```python
from build123d import *

# Parameters (mm, degrees)
SKETCH1_R           = 30
BOSS_EXTRUDE1_DEPTH = 17
SKETCH2_R           = 3.5
CUT_EXTRUDE1_DEPTH  = 16.5
SKETCH3_R           = 10
BOSS_EXTRUDE2_DEPTH = 1


with BuildPart() as part:
    # Sketch1 → Boss-Extrude1 (new body)
    with BuildSketch(Plane(origin=(0, 0, 0), x_dir=(1, 0, 0), z_dir=(0, 1, 0))):
        with Locations(Location((0, 0, 0), (0, 0, 270))):
            Circle(SKETCH1_R)
    extrude(amount=BOSS_EXTRUDE1_DEPTH)

    # Sketch2 → Cut-Extrude1 (cut)
    with BuildSketch(Plane.XY.offset(30)):
        with Locations((-16.875, 8.25)):
            Circle(SKETCH2_R)
        with BuildLine():
            Line((14.125, 11.75), (19.625, 11.75))
            ThreePointArc((19.625, 11.75), (23.125, 8.25), (19.625, 4.75))
            Line((19.625, 4.75), (14.125, 4.75))
            ThreePointArc((14.125, 4.75), (10.625, 8.25), (14.125, 11.75))
        make_face()
    extrude(amount=-CUT_EXTRUDE1_DEPTH, mode=Mode.SUBTRACT)

    # Sketch3 → Boss-Extrude2 (add)
    with BuildSketch(Plane.XZ):
        with Locations(Location((0, 0, 0), (0, 0, 270))):
            Circle(SKETCH3_R)
    extrude(amount=BOSS_EXTRUDE2_DEPTH)


solid = part.part
```
Part model, mm, in its own coordinate system. A direction names the side the tool comes from. Round coordinates to 2 decimals unless told otherwise and drop trailing zeros. Order: outer loops, then holes, each group sorted by start corner. A loop starts at its lowest first (then second) coordinate and runs counter-clockwise, first axis right, second up. Notation, with made-up numbers: M 59,85.25 L 79,85.25 A16 cw 79,107.25 Z; hole C -34,43.5 d8. An arc over 180 degrees is marked long. Answer in a Markdown table with one row per item. Add a question column.
Q1. Mould opens along X. For faces 4 (the face through (-9.76, -0.49, 2.17)), 5 (the face through (17, 4.75, 19)), 6 (the face through (0, 17, 0)) say: +X half, -X half, draft (parallel to the pull), parting line (faces both ways), or undercut.
Q2. 3-axis set-ups, long thin cutter, end or side, ignore diameter. For faces 1 (the face through (17, 11.75, 19)), 2 (the face through (0, 0, 13)), 3 (the face through (0, -1, 0)): which of +Z, -Z, +X, -X, +Y, -Y reach the whole face in a straight line?
Q3. Cut at C-C on y = 13.25. Give the cut face in (x, z).
Q4. Pin check, flat tips, straight feed: pin 1 (3 mm diameter, centred on x = -2.5, z = 22, fed in from -Y); pin 2 (1.5 mm diameter, centred on x = 19, y = 2, fed in from +Z); pin 3 (5.5 mm diameter, centred on x = -16, y = 8.5, fed in from +Z). Stop position of each tip, or through.
Q5. Wall check: L1, parallel to X at y = 8.25, z = 18.75 (3 decimals); L2, parallel to Y at x = 17.5, z = 22.5; L3, parallel to X at y = 8.25, z = 17.25 (3 decimals). Give the ranges that are in metal, low to high. Write a range as from..to.
Q6. Cut at A-A on x = 0. Give the cut face in (y, z).
Q7. Cut at B-B on z = 0. Give the cut face in (x, y).
Q8. Cut at D-D on z = -22.5. Give the cut face in (x, y).
Established:
| question | item | result |
|---|---|---|
| 1 | face 4 | parting line |
| 1 | face 5 | undercut |
| 1 | face 6 | draft |
| 2 | face 1 | +Z |
| 2 | face 2 | -Y |
| 2 | face 3 | +Z, -Z, +X, -X, -Y |
| 3 | outline | C 0,0 d60 |
| 4 | pin 1 | stops at y = 0 |
| 4 | pin 2 | stops at z = 23.81 |
| 4 | pin 3 | stops at z = 26.92 |
| 5 | L1 | x = -23.419..-20.375, -13.375..10.625, 23.125..23.419 |
| 5 | L2 | y = 0..4.75, 11.75..17 |
| 5 | L3 | x = -24.545..-20.375, -13.375..10.625, 23.125..24.545 |
| 6 | outline | M -1,-10 L 0,-10 L 0,-30 L 17,-30 L 17,30 L 0,30 L 0,10 L -1,10 Z |
| 7 | outline | M -30,0 L -10,0 L -10,-1 L 10,-1 L 10,0 L 30,0 L 30,17 L -30,17 Z |
| 8 | outline | M -19.84,0 L 19.84,0 L 19.84,17 L -19.84,17 Z |
